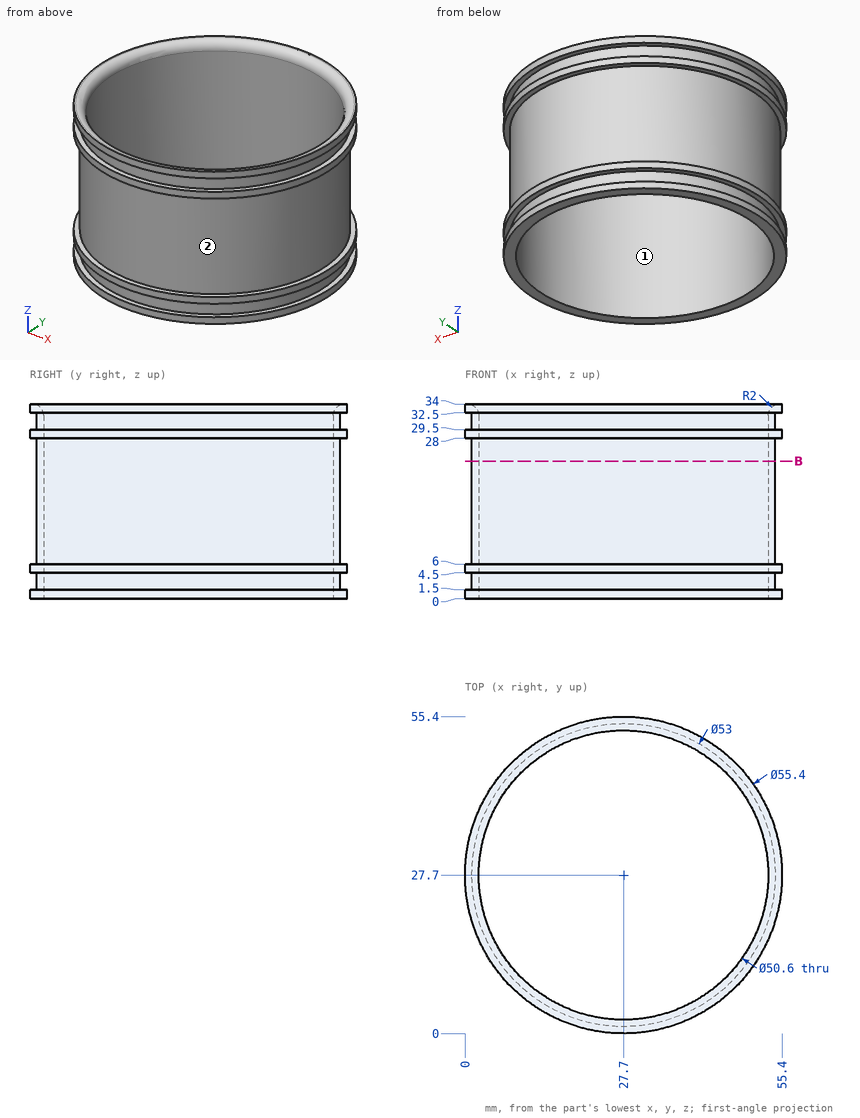
Geometry check sheet. Reference: drawing and pictorial views, mm from the part's lowest x, y, z. Give positions to 0.01 mm unless a question says otherwise; leave off trailing zeros. Write each loop counter-clockwise with the first axis right and the second up, starting at its lowest first coordinate (ties: lowest second). Pieces come first, ordered by that corner, then holes. Notation, with made-up numbers: (32.5, -10) - (74.5, -10) arc R18 ccw to (74.5, -2) - close; hole circle Ø3 at (10, 9.25). An arc over 180 degrees is marked (long way). Put each result on its own line as item: value.
Q1. Scan lines: probe 1 along Y at (x, z) = (28.5, 5.5); probe 2 along X at (y, z) = (27, 15). Record each from-to range of solid material in increasing order. Write a range as from..to.
Result:
probe 1: 0.01..2.41, 52.99..55.39
probe 2: 1.21..2.41, 52.99..54.19
Q2. Section check B-B on z = 24. Record the cut outline in (x, y), and give its area (3 significant figures).
Result:
outline: circle Ø53 at (27.7, 27.7); hole circle Ø50.6 at (27.7, 27.7)
area: 195 mm2
Q3. Depth check by flat-ended pin: P1, Ø10, axis at y = 16.5, z = 22.5, coming from the +X side; P2, Ø6, axis at x = 7.5, z = 21, coming from the +Y side; P3, Ø2, axis at y = 16.5, z = 26.5, coming from the -X side. Enter the tip coordinate at first touch or a pass-through.
Result:
P1: x = 53.46
P2: y = 47.86
P3: x = 3.24
Q4. Mould release check, pull along Y, two halves, no side actions. Record for the marked faces 1 and 2: released by +Y, released by -Y, zero draft, split by the parting line, or undercut.
Result:
face 1: undercut
face 2: split by the parting line
